Source: CAD feature listing. Evaluate the final solid. Frame: model axes, mm. A direction names the side the tool comes from. Round coordinates to 2 decimals unless told otherwise and drop trailing zeros. Loops run counter-clockwise (first coordinate to the right, second up) from the corner with the lowest first, then second, coordinate; pieces in that order, holes last.
Item 1: Section query B-B on x = -7.25. Return loops of the section in (y, z), then the cut area to 3 significant figures.
Item 2: Access query for faces 1 (the flat face through (-9.237, -3.497, 6.683)), 2 (the flat face through (-7, 2, 16.5)). Directions: +Z, -Z, +X, -X, +Y, -Y. A direction counts if a zero-diameter tool reaches every point of the face in a straight line with its end or side. Return the directions, or none.
Item 3: First-contact query: P1, Ø4.5, axis at x = -7, y = 3.5, coming from the -Z side; P2, Ø8, axis at y = -8, z = 15.5, coming from the +X side; P3, Ø4, axis at y = -6, z = 2, coming from the -X side; P4, Ø3, axis at y = 2.5, z = 8.5, coming from the -X side. Flat tips, straight axial feed; report the tip coordinate or a pass-through.
Item 4: Section query C-C on y = 5.25. Return loops of the section in (x, z).
Item 5: Section query A-A on y = 0. Return loops of the section in (x, z).
Item 6: Pull-direction query (X, two-part tool) for faces 3 (the flat face through (0, -1, 17.5)), 4 (the flat face through (5.642, 6.565, 8.858)), 5 (the flat face through (-6.18, 7.7, 6.68)); classes: released by +X, released by -X, zero draft, split by the parting line, or undercut.
Item 7: Ray query, L1, parallel to Z at x = 0.25, y = -0.25; L2, parallel to X at y = 7.25, z = 4; L3, parallel to Y at x = -3, z = 8. Return the intervals inside material, ascending.
```python
from build123d import *

# Parameters (mm, degrees)
F1_DEPTH = 16.5
F2_R     = 6.48
F3_DEPTH = 15.5
F5_DEPTH = 1
F6_DEPTH = 15.5


with BuildPart() as f1:
    # F0 (on Top) → F1 (new body)
    with BuildSketch(Plane.XY):
        Polygon((6, 8.2582915228), (-6, 8.2582915228), (-9.7082039325, -3.1543866727), (0, -10.2078097002), (9.7082039325, -3.1543866727), align=None)
    extrude(amount=F1_DEPTH)

    # F2 (on face) → F3 (cut)
    with BuildSketch(Plane.XY.offset(16.5)):
        Polygon((-7.8433001378, -3.9901700397), (-8.0901699437, -4.3299571773), (-1.6180339887, -9.0322391956), (-1.3711641828, -8.692452058), (-0.9666556856, -8.9863446841), (-0.4376489585, -8.2582293892), (-7.7188019079, -2.9681621186), (-8.247808635, -3.6962774135), align=None)
        Polygon((-6.6180339887, 6.3561784902), (-9.0901699437, -1.2522736401), (-8.6907262069, -1.3820607778), (-8.8452347041, -1.8575890359), (-7.9892838394, -2.1357043308), (-5.2081308901, 6.4238043158), (-6.0640817547, 6.7019196107), (-6.2185902519, 6.2263913526), align=None)
        Polygon((1.6180339887, -9.0322391956), (8.0901699437, -4.3299571773), (7.8433001378, -3.9901700397), (8.247808635, -3.6962774135), (7.7188019079, -2.9681621186), (0.4376489585, -8.2582293892), (0.9666556856, -8.9863446841), (1.3711641828, -8.692452058), align=None)
        Polygon((4, 8.2582915228), (-4, 8.2582915228), (-4, 7.8382915228), (-4.5, 7.8382915228), (-4.5, 6.9382915228), (4.5, 6.9382915228), (4.5, 7.8382915228), (4, 7.8382915228), align=None)
        Polygon((9.0901699437, -1.2522736401), (6.6180339887, 6.3561784902), (6.2185902519, 6.2263913526), (6.0640817547, 6.7019196107), (5.2081308901, 6.4238043158), (7.9892838394, -2.1357043308), (8.8452347041, -1.8575890359), (8.6907262069, -1.3820607778), align=None)
        Circle(F2_R)
    extrude(amount=-F3_DEPTH, mode=Mode.SUBTRACT)

    # F4 (on face) → F5 (join)
    with BuildSketch(Plane.XY.offset(16.5)):
        Polygon((6, 8.2582915228), (-6, 8.2582915228), (-9.7082039325, -3.1543866727), (0, -10.2078097002), (9.7082039325, -3.1543866727), align=None)
    extrude(amount=F5_DEPTH)

    # F2 (on face) → F6 (cut)
    with BuildSketch(Plane.XY.offset(16.5)):
        Polygon((-7.8433001378, -3.9901700397), (-8.0901699437, -4.3299571773), (-1.6180339887, -9.0322391956), (-1.3711641828, -8.692452058), (-0.9666556856, -8.9863446841), (-0.4376489585, -8.2582293892), (-7.7188019079, -2.9681621186), (-8.247808635, -3.6962774135), align=None)
        Polygon((-6.6180339887, 6.3561784902), (-9.0901699437, -1.2522736401), (-8.6907262069, -1.3820607778), (-8.8452347041, -1.8575890359), (-7.9892838394, -2.1357043308), (-5.2081308901, 6.4238043158), (-6.0640817547, 6.7019196107), (-6.2185902519, 6.2263913526), align=None)
        Polygon((1.6180339887, -9.0322391956), (8.0901699437, -4.3299571773), (7.8433001378, -3.9901700397), (8.247808635, -3.6962774135), (7.7188019079, -2.9681621186), (0.4376489585, -8.2582293892), (0.9666556856, -8.9863446841), (1.3711641828, -8.692452058), align=None)
        Polygon((4, 8.2582915228), (-4, 8.2582915228), (-4, 7.8382915228), (-4.5, 7.8382915228), (-4.5, 6.9382915228), (4.5, 6.9382915228), (4.5, 7.8382915228), (4, 7.8382915228), align=None)
        Polygon((9.0901699437, -1.2522736401), (6.6180339887, 6.3561784902), (6.2185902519, 6.2263913526), (6.0640817547, 6.7019196107), (5.2081308901, 6.4238043158), (7.9892838394, -2.1357043308), (8.8452347041, -1.8575890359), (8.6907262069, -1.3820607778), align=None)
        Circle(F2_R)
    extrude(amount=-F6_DEPTH, mode=Mode.SUBTRACT)


solid = f1.part
```
Data:
1. outline: (-4.94, 0) - (4.41, 0) - (4.41, 1) - (0.14, 1) - (0.14, 16.5) - (4.41, 16.5) - (4.41, 17.5) - (-4.94, 17.5) - (-4.94, 16.5) - (-3.31, 16.5) - (-3.31, 1) - (-4.94, 1) - close
1. area: 72.2 mm2
2. face 1: +Z, -Z, -X, -Y
2. face 2: none
3. P1: stops at z = 0
3. P2: stops at x = 8.54
3. P3: stops at x = -8.54
3. P4: stops at x = -6.97
4. outline: (-6.98, 0) - (6.98, 0) - (6.98, 1) - (5.59, 1) - (5.59, 16.5) - (6.98, 16.5) - (6.98, 17.5) - (-6.98, 17.5) - (-6.98, 16.5) - (-5.59, 16.5) - (-5.59, 1) - (-6.98, 1) - close; hole (-3.8, 1) - (3.8, 1) - (3.8, 16.5) - (-3.8, 16.5) - close
5. outline: (-8.68, 0) - (8.68, 0) - (8.68, 1) - (7.3, 1) - (7.3, 16.5) - (8.68, 16.5) - (8.68, 17.5) - (-8.68, 17.5) - (-8.68, 16.5) - (-7.3, 16.5) - (-7.3, 1) - (-8.68, 1) - close; hole (-6.48, 1) - (6.48, 1) - (6.48, 16.5) - (-6.48, 16.5) - close
6. face 3: zero draft
6. face 4: undercut
6. face 5: released by -X
7. L1: z = 0 to 1, 16.5 to 17.5
7. L2: x = -6.33 to -4.5, 4.5 to 6.33
7. L3: y = -6.4 to -5.74, 5.74 to 6.94
